Design review of the part built by this model. Coordinates are the model's own, in mm. Coordinates: 2 decimals unless noted, no trailing zeros. Write each loop counter-clockwise with the first axis right and the second up, starting at its lowest first coordinate (ties: lowest second). Pieces come first, ordered by that corner, then holes. Notation, with made-up numbers: (21.25, 9) - (56.25, 9) arc R12 ccw to (56.25, 16) - close; hole circle Ø11 at (19.25, 15). An arc over 180 degrees is marked (long way). Answer as a JSON object with one key per item and string values.
```python
from build123d import *

# Parameters (mm, degrees)
SKETCH1_W           = 10
SKETCH1_H           = 10
BOSS_EXTRUDE1_DEPTH = 204
SKETCH2_R           = 3.5
CUT_EXTRUDE1_DEPTH  = 10
LPATTERN1_COUNT     = 20
LPATTERN1_PITCH     = 10
FILLET1_R           = 5


with BuildPart() as part:
    # Sketch1 → Boss-Extrude1 (new body)
    with BuildSketch(Plane(origin=(0, 0, 0), x_dir=(0, 0, -1), z_dir=(1, 0, 0))):
        with Locations((5, 5)):
            Rectangle(SKETCH1_W, SKETCH1_H)
    extrude(amount=BOSS_EXTRUDE1_DEPTH)

    # Sketch2 → Cut-Extrude1 (cut)
    with BuildSketch(Plane(origin=(0, 10, 0), x_dir=(1, 0, 0), z_dir=(0, 1, 0))):
        with Locations(Location((7, 5, 0), (0, 0, 270))):
            Circle(SKETCH2_R)
    cut_extrude1 = extrude(amount=-CUT_EXTRUDE1_DEPTH, mode=Mode.SUBTRACT)

    # LPattern1: Cut-Extrude1 ×20
    with Locations(*[(i * LPATTERN1_PITCH, 0, 0) for i in range(1, LPATTERN1_COUNT)]):
        add(cut_extrude1, mode=Mode.SUBTRACT)

    # Fillet1
    fillet1_edges = [part.edges().sort_by_distance(p)[0] for p in [
        (0, 5, 0),
        (0, 5, -10),
        (204, 5, 0),
        (204, 5, -10),
    ]]
    fillet(fillet1_edges, radius=FILLET1_R - 0.0001)  # a hair under: the kernel refuses the full size


solid = part.part
```
(1) For pin 1 (1 mm diameter, centred on y = 2, z = -4, fed in from -X), flat-tipped, find the tip position at first contact; note if it passes through.
Solved:
{"pin 1": "stops at x = 0.03"}
(2) Take a section at A-A, the plane x = 187. Write out the cut boundary in (y, z), and give its area (3 significant figures).
Solved:
{"outline": "(0, -10) - (10, -10) - (10, -8.5) - (0, -8.5) - close; (0, -1.5) - (10, -1.5) - (10, 0) - (0, 0) - close", "area": "30.0 mm^2"}
(3) Take a section at B-B, the plane y = 3.75. Give the number of separate pieces and of enclosed holes in the cut face, and give its area (3 significant figures).
Solved:
{"separate pieces": "1", "enclosed holes": "20", "area": "1,250 mm^2"}
(4) To check wall thickness, follow line 1 (Z direction, x = 37, y = 2.5); line 2 (Z direction, x = 78.5, y = 7); line 3 (X direction, y = 9.25, z = -1). State the ranges of each line that lie inside material, in increasing order. Write a range as from..to.
Solved:
{"line 1": "z = -10..-8.5, -1.5..0", "line 2": "z = -10..-8.16, -1.84..0", "line 3": "x = 2..202"}
(5) The part is to be moulded in two halves that separate along X. For faces 1 (the face through (2, 5, -1)), 2 (the face through (101, 10, -5)), 3 (the face through (203, 5, -8)), 4 (the face through (20.47, 5.07, -5.46)), say which applies: pulls with the +X half, pulls with the -X half, needs draft (parallel to the pull), parting line crosses it, or undercut.
Solved:
{"face 1": "pulls with the -X half", "face 2": "needs draft", "face 3": "pulls with the +X half", "face 4": "undercut"}
